For this review, take the finished solid that the model builds, in its own axes (mm). A direction names the side the tool comes from. Round coordinates to 2 decimals unless told otherwise and drop trailing zeros. Write each loop counter-clockwise with the first axis right and the second up, starting at its lowest first coordinate (ties: lowest second). Pieces come first, ordered by that corner, then holes. Notation, with made-up numbers: (88, 80) - (101, 80) arc R20 ccw to (101, 94) - close; hole circle Ø6 at (88, 60.5). An arc over 180 degrees is marked (long way). One line per item, written item: value. Start each with the question number.
Q1. Clearance check with flat-ended pins moving along their axes: pin 1 Ø0.9 at (x, z) = (149.5, 2) entering from -Y; pin 2 Ø1.5 at (y, z) = (202, 1) entering from -X. State where each tip first meets the part, or that it passes through.
Q2. Add section C-C on x = 157.5. Write out the cut boundary in (y, z).
Q3. Tool access review of faces 1 (the face through (156, 205, 0)), 2 (the face through (153.842, 201, 1)), 3 (the face through (152.592, 207, 1)): name each direction out of +Z, -Z, +X, -X, +Y, -Y from which nothing blocks a thin tool from reaching the whole face with its end or side.
Q4. For probe 1 along X at (y, z) = (208.25, 1.05); probe 2 along Y at (x, z) = (149.5, 0.2); probe 3 along Y at (x, z) = (153, 0.6), list the stretches that pass through material, from the lowest coordinate up.
Q5. Add section D-D on y = 197.25. Write out the cut boundary in (x, z).
Q6. Mouldability with a two-part tool opening along Y and no side actions: class faces 4 (the face through (154, 211.824, 1)), 5 (the face through (155.092, 207, 1)), 6 (the face through (162.842, 205, 1)) as +Y half, -Y half, draft (parallel to the pull), parting line (faces both ways), or undercut.
Q7. Add section A-A on z = 2.35. Write out the cut boundary in (x, y).
Q8. Add section B-B on x = 147.25. Write out the cut boundary in (y, z).
```python
from build123d import *

# Parameters (mm, degrees)
MODEL_R                 = 1.5
SALIENTE_EXTRUIR1_DEPTH = 3


with BuildPart() as part:
    # Model → Saliente-Extruir1 (new body)
    with BuildSketch(Plane.XY):
        with BuildLine():
            Line((149.34213351, 211.823953209), (158.34213351, 211.823953209))
            Line((158.34213351, 211.823953209), (162.84213351, 211.823953209))
            Line((162.84213351, 211.823953209), (162.84213351, 198.323953209))
            ThreePointArc((162.84213351, 198.323953209), (158.34213351, 193.823953209), (153.84213351, 198.323953209))
            Line((153.84213351, 198.323953209), (153.84213351, 202.823953209))
            Line((153.84213351, 202.823953209), (149.34213351, 202.823953209))
            ThreePointArc((149.34213351, 202.823953209), (146.160152994, 204.141972694), (144.84213351, 207.323953209))
            Line((144.84213351, 207.323953209), (144.84213351, 211.823953209))
            Line((144.84213351, 211.823953209), (149.34213351, 211.823953209))
        make_face()
        with Locations((158.34213351, 198.323953209)):
            Circle(MODEL_R, mode=Mode.SUBTRACT)
        with BuildLine():
            Line((151.84213351, 205.698953209), (146.84213351, 205.698953209))
            ThreePointArc((146.84213351, 205.698953209), (146.311803424, 205.918623123), (146.09213351, 206.448953209))
            Line((146.09213351, 206.448953209), (146.09213351, 208.198953209))
            ThreePointArc((146.09213351, 208.198953209), (146.311803424, 208.729283295), (146.84213351, 208.948953209))
            Line((146.84213351, 208.948953209), (151.84213351, 208.948953209))
            ThreePointArc((151.84213351, 208.948953209), (152.372463595, 208.729283295), (152.59213351, 208.198953209))
            Line((152.59213351, 208.198953209), (152.59213351, 206.448953209))
            ThreePointArc((152.59213351, 206.448953209), (152.372463595, 205.918623123), (151.84213351, 205.698953209))
        make_face(mode=Mode.SUBTRACT)
        with BuildLine():
            Line((160.84213351, 205.698953209), (155.84213351, 205.698953209))
            ThreePointArc((155.84213351, 205.698953209), (155.311803424, 205.918623123), (155.09213351, 206.448953209))
            Line((155.09213351, 206.448953209), (155.09213351, 208.198953209))
            ThreePointArc((155.09213351, 208.198953209), (155.311803424, 208.729283295), (155.84213351, 208.948953209))
            Line((155.84213351, 208.948953209), (160.84213351, 208.948953209))
            ThreePointArc((160.84213351, 208.948953209), (161.372463595, 208.729283295), (161.59213351, 208.198953209))
            Line((161.59213351, 208.198953209), (161.59213351, 206.448953209))
            ThreePointArc((161.59213351, 206.448953209), (161.372463595, 205.918623123), (160.84213351, 205.698953209))
        make_face(mode=Mode.SUBTRACT)
    extrude(amount=SALIENTE_EXTRUIR1_DEPTH)


solid = part.part
```
Result set:
1. pin 1: stops at y = 202.82
1. pin 2: stops at x = 153.84
2. outline: (193.9, 0) - (197.08, 0) - (197.08, 3) - (193.9, 3) - close; (199.57, 0) - (205.7, 0) - (205.7, 3) - (199.57, 3) - close; (208.95, 0) - (211.82, 0) - (211.82, 3) - (208.95, 3) - close
3. face 1: -Z, +X, -X, +Y, -Y
3. face 2: +Z, -Z, -X, -Y
3. face 3: +Z, -Z
4. probe 1: x = 144.84 to 146.09, 152.59 to 155.09, 161.59 to 162.84
4. probe 2: y = 202.82 to 205.7, 208.95 to 211.82
4. probe 3: y = 202.82 to 211.82
5. outline: (153.97, 0) - (157.29, 0) - (157.29, 3) - (153.97, 3) - close; (159.39, 0) - (162.71, 0) - (162.71, 3) - (159.39, 3) - close
6. face 4: +Y half
6. face 5: undercut
6. face 6: draft
7. outline: (144.84, 207.32) arc R4.5 ccw to (149.34, 202.82) - (153.84, 202.82) - (153.84, 198.32) arc R4.5 ccw to (162.84, 198.32) - (162.84, 211.82) - (144.84, 211.82) - close; hole (146.09, 206.45) arc R0.75 ccw to (146.84, 205.7) - (151.84, 205.7) arc R0.75 ccw to (152.59, 206.45) - (152.59, 208.2) arc R0.75 ccw to (151.84, 208.95) - (146.84, 208.95) arc R0.75 ccw to (146.09, 208.2) - close; hole (155.09, 206.45) arc R0.75 ccw to (155.84, 205.7) - (160.84, 205.7) arc R0.75 ccw to (161.59, 206.45) - (161.59, 208.2) arc R0.75 ccw to (160.84, 208.95) - (155.84, 208.95) arc R0.75 ccw to (155.09, 208.2) - close; hole circle Ø3 at (158.34, 198.32)
8. outline: (203.34, 0) - (205.7, 0) - (205.7, 3) - (203.34, 3) - close; (208.95, 0) - (211.82, 0) - (211.82, 3) - (208.95, 3) - close
